```python
from build123d import *

# Parameters (mm, degrees)
F0_W     = 100
F0_H     = 45
F1_DEPTH = 15
F3_DEPTH = 30
F5_DEPTH = 33
F7_DEPTH = 15


with BuildPart() as f1:
    # F0 (on Top) → F1 (new body)
    with BuildSketch(Plane.XY):
        with Locations((-2.304982, -13.08857)):
            Rectangle(F0_W, F0_H)
    extrude(amount=F1_DEPTH)

    # F2 (on face) → F3 (join)
    with BuildSketch(Plane.XY.offset(15)):
        Polygon((2.695018, -35.58857), (2.695018, 9.41143), (-12.304982, 9.41143), (-12.304982, -20.58857), (-52.304982, -20.58857), (-52.304982, -35.58857), (-12.304982, -35.58857), align=None)
    extrude(amount=F3_DEPTH)

    # F4 (on face) → F5 (join)
    with BuildSketch(Plane(origin=(0, 9.41143, 0), x_dir=(-1, 0, 0), z_dir=(0, 1, 0))):
        Polygon((52.304982, 15), (12.304982, 45), (12.304982, 15), align=None)
    extrude(amount=-F5_DEPTH)

    # F6 (on face) → F7 (join)
    with BuildSketch(Plane.XZ.offset(35.58857)):
        Polygon((47.695018, 15), (2.695018, 45), (2.695018, 15), align=None)
    extrude(amount=-F7_DEPTH)


solid = f1.part
```
Can you work these out from the model? Positions are in its coordinate system, mm. A direction names the side the tool comes from. Coordinates: 2 decimals unless noted, no trailing zeros. Loops run counter-clockwise (first coordinate to the right, second up) from the corner with the lowest first, then second, coordinate; pieces in that order, holes last. Notation, with made-up numbers: (-29, 86) - (-2, 86) arc R28 cw to (-2, 122) - close; hole circle Ø4 at (56, 52). An arc over 180 degrees is marked (long way). Use a Markdown table: item, result.
Item 1: I want a section at C-C on x = -17.5. Please give me the cut outline in (y, z).
Numbers:
| item | result |
|---|---|
| outline | (-35.59, 0) - (9.41, 0) - (9.41, 41.1) - (-20.59, 41.1) - (-20.59, 45) - (-35.59, 45) - close |
Item 2: For faces 1 (the face through (2.695, -6, 30)), 2 (the face through (25.51, -28.19, 29.79)), 3 (the face through (-41, -20.589, 36)), which set-ups out of +Z, -Z, +X, -X, +Y, -Y let a thin tool reach every point of the face, with its end or its side?
Numbers:
| item | result |
|---|---|
| face 1 | +Z, +X, +Y |
| face 2 | +Z, +X, +Y, -Y |
| face 3 | +Z, -X, +Y |
Item 3: If I drill on probe 1 along Y at (x, z) = (11, 34); probe 2 along Z at (x, y) = (10, 5); probe 3 along X at (y, z) = (-1, 27.5), over which ranges is the centre line in solid material (lowest first)? Write a range as from..to.
Numbers:
| item | result |
|---|---|
| probe 1 | y = -35.59..-20.59 |
| probe 2 | z = 0..15 |
| probe 3 | x = -35.64..2.7 |
Item 4: I want a section at D-D on z = 40. Please give me the cut outline in (x, y), and give its area (3 significant figures).
Numbers:
| item | result |
|---|---|
| outline | (-52.3, -35.59) - (10.2, -35.59) - (10.2, -20.59) - (2.7, -20.59) - (2.7, 9.41) - (-18.97, 9.41) - (-18.97, -20.59) - (-52.3, -20.59) - close |
| area | 1,590 mm2 |
Item 5: I want a section at A-A on y = -16.5. Please give me the cut outline in (x, z).
Numbers:
| item | result |
|---|---|
| outline | (-52.3, 0) - (47.7, 0) - (47.7, 15) - (2.7, 15) - (2.7, 45) - (-12.3, 45) - (-52.3, 15) - close |
Item 6: Will these pins go through, and if not, where does the flat tip stop? pin 1 (3 mm diameter, centred on x = 6, y = -11, fed in from +Z); pin 2 (4 mm diameter, centred on x = -22.5, y = 4, fed in from +Z); pin 3 (24 mm diameter, centred on x = 16, z = 36.5, fed in from +Y).
Numbers:
| item | result |
|---|---|
| pin 1 | stops at z = 15 |
| pin 2 | stops at z = 38.85 |
| pin 3 | stops at y = -20.59 |
Item 7: I want a section at B-B on z = 33. Please give me the cut outline in (x, y), and give its area (4 significant figures).
Numbers:
| item | result |
|---|---|
| outline | (-52.3, -35.59) - (20.7, -35.59) - (20.7, -20.59) - (2.7, -20.59) - (2.7, 9.41) - (-28.3, 9.41) - (-28.3, -20.59) - (-52.3, -20.59) - close |
| area | 2,025 mm2 |
